Verification items for the finished model (mm, model axes). Round coordinates to 2 decimals unless told otherwise and drop trailing zeros. Order: outer loops, then holes, each group sorted by start corner. A loop starts at its lowest first (then second) coordinate and runs counter-clockwise, first axis right, second up. Notation, with made-up numbers: (57.25, -18.5) -> (63.25, -18.5) arc R25 cw to (63.25, 1.5) -> close; hole circle Ø6 at (87.5, -31.75). An arc over 180 degrees is marked (long way). Put each result on its own line as item: value.
from build123d import *

# Parameters (mm, degrees)
SKETCH_1_W          = 73
SKETCH_1_H          = 30
EXTRUDE_1_DEPTH     = 8
SKETCH_2_R          = 1.5
CUT_EXTRUDE_1_DEPTH = 45


with BuildPart() as part:
    # 草图1 → 凸台-拉伸1 (new body)
    with BuildSketch(Plane(origin=(0, 0, 0), x_dir=(1, 0, 0), z_dir=(0, 1, 0))):
        Rectangle(SKETCH_1_W, SKETCH_1_H)
    extrude(amount=EXTRUDE_1_DEPTH)

    # 草图2 → 切除-拉伸1 (cut, symmetric)
    with BuildSketch(Plane(origin=(59.282070169, -28, -16.5), x_dir=(1, 0, 0), z_dir=(0, -1, 0))):
        with Locations((-28.282070169, 14)):
            Circle(SKETCH_2_R)
        with Locations((-90.282070169, 14)):
            Circle(SKETCH_2_R)
        with Locations((-90.282070169, 26)):
            Circle(SKETCH_2_R)
        with Locations((-28.282070169, 26)):
            Circle(SKETCH_2_R)
    extrude(amount=CUT_EXTRUDE_1_DEPTH, both=True, mode=Mode.SUBTRACT)


solid = part.part
Item 1: Material ranges on L1, parallel to Z at x = -31, y = 5.25; L2, parallel to X at y = 1.75, z = 10.75; L3, parallel to X at y = 1.5, z = -1.75, recorded low to high. Write a range as [from, to].
Check sheet entries:
L1: z = [-15, -4], [-1, 8], [11, 15]
L2: x = [-36.5, -31.83], [-30.17, 30.17], [31.83, 36.5]
L3: x = [-36.5, -32.3], [-29.7, 29.7], [32.3, 36.5]
Item 2: Section check A-A on x = -31. Record the boundary of the cut face in (y, z), then the cut area to 3 significant figures.
Check sheet entries:
outline: (0, -15) -> (8, -15) -> (8, -4) -> (0, -4) -> close; (0, -1) -> (8, -1) -> (8, 8) -> (0, 8) -> close; (0, 11) -> (8, 11) -> (8, 15) -> (0, 15) -> close
area: 192 mm^2
Item 3: Release check for a two-part mould opening along Z. For faces 1 (the cylindrical face through (-32.2, 3.9, 8.6)), 2 (the flat face through (-36.5, 4, 0)), 3 (the flat face through (-1, 4, -15)) record: +Z half, -Z half, draft (parallel to the pull), parting line (faces both ways), or undercut.
Check sheet entries:
face 1: undercut
face 2: draft
face 3: -Z half
Item 4: Section check B-B on z = 9.5. Record the boundary of the cut face in (x, y), then the cut area to 3 significant figures.
Check sheet entries:
outline: (-36.5, 0) -> (-32.5, 0) -> (-32.5, 8) -> (-36.5, 8) -> close; (-29.5, 0) -> (29.5, 0) -> (29.5, 8) -> (-29.5, 8) -> close; (32.5, 0) -> (36.5, 0) -> (36.5, 8) -> (32.5, 8) -> close
area: 536 mm^2
Item 5: Gauge pin test, flat ends, axial feed: pin 1 Ø3 at (x, z) = (13.5, 4.5) entering from -Y; pin 2 Ø2.5 at (x, z) = (-31, 9.5) entering from -Y. Record the tip position at first contact, or that the pin passes through.
Check sheet entries:
pin 1: stops at y = 0
pin 2: passes through
